Job drawing, mm, ordinate dimensions from the low corner. One solid piece. A direction names the side the tool comes from. Coordinates: 2 decimals unless noted, no trailing zeros. Loops run counter-clockwise (first coordinate to the right, second up) from the corner with the lowest first, then second, coordinate; pieces in that order, holes last. Notation, with made-up numbers: (37, -0.75) - (47, -0.75) arc R24 cw to (47, 12.25) - close; hole circle Ø7 at (29, 70). An arc over 180 degrees is marked (long way). One line per question, with ' | ' between items. Start each with the question number.
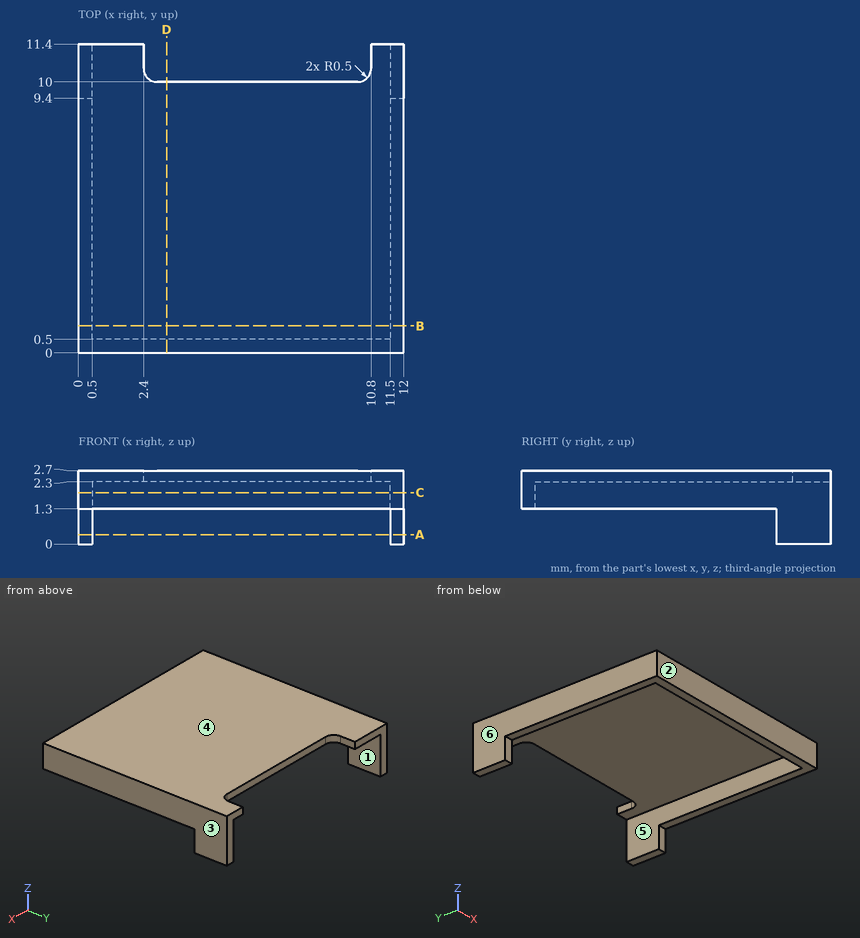
1) Pin check, flat tip, straight feed: pin 1 Ø1 at (x, y) = (8.5, 9) entering from -Z. Stop position of the tip, or through.
2) Tool access for the marked faces 1 and 2: list every direction of +Z, -Z, +X, -X, +Y, -Y with a clear straight run to the whole face (end or side of a thin tool).
3) Band-saw the part on C-C on z = 1.9. List the corners of the cut face in (x, y), then the cut area to 3 significant figures.
4) Band-saw the part on B-B on y = 1. List the corners of the cut face in (x, z).
5) Wall check: line 1 along X through (y, z) = (2.25, 1.4); line 2 along Z through (x, y) = (1.5, 4.75); line 3 along Y through (x, z) = (5.75, 2.2). Give the ranges that are in metal, low to high. Write a range as [from, to].
6) Mould opens along X. For the marked faces 3, 4, 5 and 6 say: +X half, -X half, draft (parallel to the pull), parting line (faces both ways), or undercut.
7) Band-saw the part on D-D on x = 3.25. List the corners of the cut face in (y, z), then the cut area to 3 significant figures.
8) Band-saw the part on A-A on z = 0.35. List the corners of the cut face in (x, y), then the cut area to 3 significant figures.
Values found:
1) pin 1: z = 2.3
2) face 1: -Z, +Y | face 2: +Z, -Z, +X, -X, -Y
3) outline: (0, 0) - (12, 0) - (12, 11.4) - (11.5, 11.4) - (11.5, 0.5) - (0.5, 0.5) - (0.5, 11.4) - (0, 11.4) - close | area: 16.9 mm²
4) outline: (0, 1.3) - (0.5, 1.3) - (0.5, 2.3) - (11.5, 2.3) - (11.5, 1.3) - (12, 1.3) - (12, 2.7) - (0, 2.7) - close
5) line 1: [0, 0.5], [11.5, 12] | line 2: [2.3, 2.7] | line 3: [0, 0.5]
6) face 3: +X half | face 4: draft | face 5: undercut | face 6: -X half
7) outline: (0, 1.3) - (0.5, 1.3) - (0.5, 2.3) - (10, 2.3) - (10, 2.7) - (0, 2.7) - close | area: 4.50 mm²
8) outline: (0, 9.4) - (0.5, 9.4) - (0.5, 11.4) - (0, 11.4) - close; (11.5, 9.4) - (12, 9.4) - (12, 11.4) - (11.5, 11.4) - close | area: 2.00 mm²
